```python
from build123d import *

# Parameters (mm, degrees)
ESBO_O1_R                = 12.5
RESSALTO_EXTRUS_O1_DEPTH = 21
ESBO_O2_R                = 3.5
RESSALTO_EXTRUS_O2_DEPTH = 2.5
FILETE1_R                = 1
ESBO_O3_R                = 2
RESSALTO_EXTRUS_O3_DEPTH = 8
ESBO_O4_R                = 1.25
CORTE_EXTRUS_O1_DEPTH    = 10


with BuildPart() as part:
    # Esboço1 → Ressalto-extrusão1 (new body)
    with BuildSketch(Plane.XY):
        with Locations(Location((0, 0, 0), (0, 0, 180))):
            Circle(ESBO_O1_R)
    extrude(amount=RESSALTO_EXTRUS_O1_DEPTH)

    # Esboço2 → Ressalto-extrusão2 (add)
    with BuildSketch(Plane.XY.offset(21)):
        Circle(ESBO_O2_R)
    extrude(amount=RESSALTO_EXTRUS_O2_DEPTH)

    # Filete1
    filete1_edges = [part.edges().sort_by_distance(p)[0] for p in [
        (12.5, 0, 0),
        (12.5, 0, 21),
    ]]
    fillet(filete1_edges, radius=FILETE1_R)

    # Esboço3 → Ressalto-extrusão3 (add)
    with BuildSketch(Plane.XY.offset(23.5)):
        Circle(ESBO_O3_R)
    extrude(amount=RESSALTO_EXTRUS_O3_DEPTH)

    # Esboço4 → Corte-extrusão1 (cut)
    with BuildSketch(Plane.XY.offset(21)):
        with Locations((0, 8.5)):
            Circle(ESBO_O4_R)
        with Locations((0, -8.5)):
            Circle(ESBO_O4_R)
    extrude(amount=-CORTE_EXTRUS_O1_DEPTH, mode=Mode.SUBTRACT)


solid = part.part
```
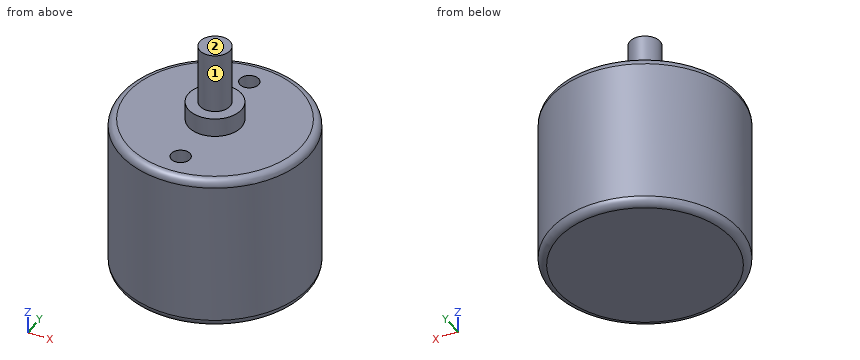
Work out the finished part from the listing and answer in its coordinate system (mm). Face numbers are marked on the shaded views. A direction names the side the tool comes from. Give positions to 0.01 mm unless a question says otherwise; leave off trailing zeros. Loops run counter-clockwise (first coordinate to the right, second up) from the corner with the lowest first, then second, coordinate; pieces in that order, holes last. Notation, with made-up numbers: (69.25, 81) -> (81.25, 81) arc R22 ccw to (81.25, 94) -> close; hole circle Ø4 at (-4, 81.5). An arc over 180 degrees is marked (long way). Write item = value, one per line. Start each with the question number.
(1) Find section B-B on x = 0. Give the vertices of the cut face in (y, z).
(2) Find section D-D on z = 9. Give the vertices of the cut face in (x, y), and give its area (3 significant figures).
(3) Which of the six approach directions +Z, -Z, +X, -X, +Y, -Y give full straight-line access (tool end or side, diameter ignored) to the marked faces 1 and 2?
(4) Find section A-A on y = 0. Give the vertices of the cut face in (x, z), and give its area (3 significant figures).
(5) Find section C-C on z = 29. Give the vertices of the cut face in (x, y), and give its area (3 significant figures).
(6) Find the intervals of material crossed by probe 1 along Y at (x, z) = (0, 13.75); probe 2 along Z at (x, y) = (6, -7.5); probe 3 along Z at (x, y) = (-1.5, 2.75), in increasing order. Write a range as from..to.
(7) Given pin 1 Ø4 at (y, z) = (2.5, 16.5) entering from +X; pin 2 Ø2 at (x, y) = (0, -8) entering from +Z; pin 3 Ø8 at (y, z) = (-7, 16.5) entering from -X; pin 4 Ø1.5 at (y, z) = (5.5, 22.5) entering from -X, each flat-ended and moving along its own axis, determine where each tip first touches the part or whether it passes through.
From the geometry:
q1.outline = (-12.5, 1) arc R1 ccw to (-11.5, 0) -> (11.5, 0) arc R1 ccw to (12.5, 1) -> (12.5, 20) arc R1 ccw to (11.5, 21) -> (9.75, 21) -> (9.75, 11) -> (7.25, 11) -> (7.25, 21) -> (3.5, 21) -> (3.5, 23.5) -> (2, 23.5) -> (2, 31.5) -> (-2, 31.5) -> (-2, 23.5) -> (-3.5, 23.5) -> (-3.5, 21) -> (-7.25, 21) -> (-7.25, 11) -> (-9.75, 11) -> (-9.75, 21) -> (-11.5, 21) arc R1 ccw to (-12.5, 20) -> close
q2.outline = circle Ø25 at (0, 0)
q2.area = 491 mm^2
q3.face_1 = +Z
q3.face_2 = +Z, +X, -X, +Y, -Y
q4.outline = (-12.5, 1) arc R1 ccw to (-11.5, 0) -> (11.5, 0) arc R1 ccw to (12.5, 1) -> (12.5, 20) arc R1 ccw to (11.5, 21) -> (3.5, 21) -> (3.5, 23.5) -> (2, 23.5) -> (2, 31.5) -> (-2, 31.5) -> (-2, 23.5) -> (-3.5, 23.5) -> (-3.5, 21) -> (-11.5, 21) arc R1 ccw to (-12.5, 20) -> close
q4.area = 574 mm^2
q5.outline = circle Ø4 at (0, 0)
q5.area = 12.6 mm^2
q6.probe_1 = -12.5..-9.75, -7.25..7.25, 9.75..12.5
q6.probe_2 = 0..21
q6.probe_3 = 0..23.5
q7.pin_1 = 12.49
q7.pin_2 = 21
q7.pin_3 = -12.13
q7.pin_4 = through
